Here's how the part is built. I have some questions about the finished solid (model axes, mm). Give positions to 0.01 mm unless a question says otherwise; leave off trailing zeros. Loops run counter-clockwise (first coordinate to the right, second up) from the corner with the lowest first, then second, coordinate; pieces in that order, holes last. Notation, with made-up numbers: (81.5, -17.5) - (116.5, -17.5) arc R27 cw to (116.5, 15.5) - close; hole circle Ø9 at (30, 51). An arc over 180 degrees is marked (long way). Put each result on its own line as item: value. Start each with the question number.
from build123d import *

# Parameters (mm, degrees)
SKETCH_1_R               = 9
SKETCH_1_R_2             = 6.25
EXTRUDE_1_DEPTH          = 150
SKETCH_2_R               = 1.75
CUT_EXTRUDE_1_DEPTH      = 10
CUT_EXTRUDE_1_DEPTH_BACK = 10
SKETCH_3_R               = 1.75
CUT_EXTRUDE_2_DEPTH      = 10.0000001
CUT_EXTRUDE_2_DEPTH_BACK = 10.0000001


with BuildPart() as part:
    # ｽｹｯﾁ1 → ﾎﾞｽ - 押し出し1 (new body)
    with BuildSketch(Plane.XY):
        Circle(SKETCH_1_R)
        Circle(SKETCH_1_R_2, mode=Mode.SUBTRACT)
    extrude(amount=EXTRUDE_1_DEPTH)

    # ｽｹｯﾁ2 → ｶｯﾄ - 押し出し1 (cut, two sides)
    with BuildSketch(Plane(origin=(0, 0, 0), x_dir=(0, 0, -1), z_dir=(1, 0, 0))) as cut_extrude_1_sk:
        with Locations((-7.5, 0)):
            Circle(SKETCH_2_R)
        with Locations((-142.5, 0)):
            Circle(SKETCH_2_R)
        with Locations((-110, 0)):
            Circle(SKETCH_2_R)
    extrude(amount=CUT_EXTRUDE_1_DEPTH, mode=Mode.SUBTRACT)
    extrude(cut_extrude_1_sk.sketch, amount=-CUT_EXTRUDE_1_DEPTH_BACK, mode=Mode.SUBTRACT)

    # ｽｹｯﾁ3 → ｶｯﾄ - 押し出し2 (cut, two sides)
    with BuildSketch(Plane(origin=(0, 0, 0), x_dir=(1, 0, 0), z_dir=(0, 1, 0))) as cut_extrude_2_sk:
        with Locations((0, -45)):
            Circle(SKETCH_3_R)
    extrude(amount=CUT_EXTRUDE_2_DEPTH, mode=Mode.SUBTRACT)
    extrude(cut_extrude_2_sk.sketch, amount=-CUT_EXTRUDE_2_DEPTH_BACK, mode=Mode.SUBTRACT)


solid = part.part
1) Suppose I cut it at C-C on x = 7.75. Please give me the cut outline in (y, z).
2) Thinking about a two-plate mould opening in Y: for faces 1 (the cylindrical face through (8.584, 2.703, 73.95)), 2 (the flat face through (-6.13, -1.87, 0)), 3 (the cylindrical face through (5.96, 1.88, 73.95)), which applies, pulls with the +Y half, pulls with the -Y half, needs draft (parallel to the pull), parting line crosses it, or undercut?
3) I'm going to push flat-ended pins straight in: P1, Ø4, axis at y = 0, z = 7.5, coming from the -X side; P2, Ø1, axis at x = -2.5, z = 95.5, coming from the -Y side; P3, Ø6, axis at x = 4.5, z = 37.5, coming from the -Y side; P4, Ø1.5, axis at x = -4, z = 43, coming from the +Y side. Where does each tip first touch, or does it pass through?
4) Suppose I cut it at A-A on x = -3. Please give me the cut outline in (y, z), plus the area to 3 significant figures.
5) Suppose I cut it at D-D on z = 62. Please give me the cut outline in (x, y), plus the area to 3 significant figures.
6) I need wall thicknesses on line 1 (Z direction, x = 8.15, y = 0); line 2 (Z direction, x = -6.5, y = -1.25); line 3 (Y direction, x = 0.25, z = 87.5) (3 decimals). Which ranges of each line are inside material? Lowest first, please.
7) Suppose I cut it at B-B on z = 110. Please give me the cut outline in (x, y).
Ans:
1. outline: (-4.58, 0) - (4.58, 0) - (4.58, 150) - (-4.58, 150) - close; hole circle Ø3.5 at (0, 7.5); hole circle Ø3.5 at (0, 110); hole circle Ø3.5 at (0, 142.5)
2. face 1: parting line crosses it
2. face 2: needs draft
2. face 3: undercut
3. P1: stops at x = -9
3. P2: stops at y = -8.77
3. P3: stops at y = -8.87
3. P4: stops at y = 8.39
4. outline: (-8.49, 0) - (-5.48, 0) - (-5.48, 150) - (-8.49, 150) - close; (5.48, 0) - (8.49, 0) - (8.49, 150) - (5.48, 150) - close
4. area: 901 mm²
5. outline: circle Ø18 at (0, 0); hole circle Ø12.5 at (0, 0)
5. area: 132 mm²
6. line 1: z = 0 to 5.75, 9.25 to 108.25, 111.75 to 140.75, 144.25 to 150
6. line 2: z = 0 to 6.28, 8.72 to 108.78, 111.22 to 141.28, 143.72 to 150
6. line 3: y = -8.997 to -6.245, 6.245 to 8.997
7. outline: (-8.83, -1.75) arc R9 ccw to (8.83, -1.75) - (6, -1.75) arc R6.25 cw to (-6, -1.75) - close; (-8.83, 1.75) - (-6, 1.75) arc R6.25 cw to (6, 1.75) - (8.83, 1.75) arc R9 ccw to start
